The model under review builds one solid part; all positions refer to its coordinate system, in mm. A direction names the side the tool comes from. Give positions to 0.01 mm unless a question says otherwise; leave off trailing zeros. Loops run counter-clockwise (first coordinate to the right, second up) from the corner with the lowest first, then second, coordinate; pieces in that order, holes last. Notation, with made-up numbers: (62, -18.5) -> (99, -18.5) arc R20 cw to (99, 18.5) -> close; hole circle Ø8 at (2.5, -12.75). An arc over 180 degrees is marked (long way). Write each question's results on one line, items separated by ' | '. Start each with the question number.
Q1. Insertion check: pin 1 Ø15 at (y, z) = (-9.5, 33.5) entering from -X; pin 2 Ø12.5 at (x, y) = (41, -12) entering from +Z; pin 3 Ø8 at (y, z) = (7, 55.5) entering from +X; pin 4 Ø1.5 at (x, z) = (-34, 51) entering from -Y. Each pin has a flat end and moves straight along its axis. Give the tip position at first contact, or say it passes through.
Q2. Wall thickness on L1, parallel to X at y = -10, z = 47; L2, parallel to Z at x = -38.5, y = 4.5; L3, parallel to Y at x = -29, z = 59: over which ranges is each line inside the solid? List them lowest first. Write a range as [from, to].
Q3. Machinability: for faces 1 (the face through (-31.75, 0, 39)), 2 (the face through (-19.05, 0, 38)), 3 (the face through (-57.073, -0.557, 6.261)), which of the approach directions +Z, -Z, +X, -X, +Y, -Y give a long, thin tool a straight path to every point of the face, cutting with its end or side? Answer none if there is none.
Q4. We need section A-A (z = 34). Write out the cut boundary in (x, y).
Q5. We need section D-D (y = -7.5). Write out the cut boundary in (x, z).
Q6. We need section C-C (x = 14). Write out the cut boundary in (y, z).
Q7. Mouldability with a two-part tool opening along Y and no side actions: class faces 4 (the face through (41, 0, 12.7)), 5 (the face through (0, 25.4, 11)), 6 (the face through (25.489, -0.251, 52.073)) as released by +Y, released by -Y, zero draft, split by the parting line, or undercut.
Q8. We need section B-B (y = 4.5). Write out the cut boundary in (x, z), plus the area to 3 significant figures.
from build123d import *

# Parameters (mm, degrees)
F1_DEPTH = 25.4
F3_DEPTH = 63.501
F5_DEPTH = 12.7


with BuildPart() as f1:
    # F0 (on Front) → F1 (new body, symmetric)
    with BuildSketch(Plane.XZ):
        Polygon((-31.75, 0), (0, 0), (31.75, 0), (31.75, 63.5), (19.05, 63.5), (19.05, 12.7), (0, 12.7), (-19.05, 12.7), (-19.05, 63.5), (-31.75, 63.5), align=None)
    extrude(amount=F1_DEPTH, both=True)

    # F2 (on face) → F3 (cut, through all)
    with BuildSketch(Plane.YZ.offset(31.75)):
        with BuildLine():
            ThreePointArc((-11.43, 63.5), (0, 52.07), (11.43, 63.5))
            Line((11.43, 63.5), (-11.43, 63.5))
        make_face()
    extrude(amount=-F3_DEPTH, mode=Mode.SUBTRACT)

    # F4 (on face) → F5 (join)
    with BuildSketch(Plane(origin=(0, 0, 0), x_dir=(1, 0, 0), z_dir=(0, 0, -1))):
        with BuildLine():
            ThreePointArc((-31.75, -25.3289327497), (-13.8397398924, -17.9102601076), (-6.4210672503, 0))
            ThreePointArc((-6.4210672503, 0), (-13.8397398924, 17.9102601076), (-31.75, 25.3289327497))
            Line((-31.75, 25.3289327497), (-31.75, -25.3289327497))
        make_face()
        with BuildLine():
            Line((-31.75, -25.3289327497), (-31.75, 25.3289327497))
            ThreePointArc((-31.75, 25.3289327497), (-57.0789327497, 0), (-31.75, -25.3289327497))
        make_face()
        with BuildLine():
            ThreePointArc((57.0789327497, 0), (49.6602601076, 17.9102601076), (31.75, 25.3289327497))
            Line((31.75, 25.3289327497), (31.75, -25.3289327497))
            ThreePointArc((31.75, -25.3289327497), (49.6602601076, -17.9102601076), (57.0789327497, 0))
        make_face()
    extrude(amount=-F5_DEPTH)


solid = f1.part
Output:
1) pin 1: x = -31.75 | pin 2: z = 12.7 | pin 3: x = 31.75 | pin 4: through
2) L1: [-31.75, -19.05], [19.05, 31.75] | L2: [0, 12.7] | L3: [-25.4, -10.51], [10.51, 25.4]
3) face 1: +Z, -X, +Y, -Y | face 2: +Z, +Y, -Y | face 3: +Z, -Z, -X
4) outline: (-31.75, -25.4) -> (-19.05, -25.4) -> (-19.05, 25.4) -> (-31.75, 25.4) -> close; (19.05, -25.4) -> (31.75, -25.4) -> (31.75, 25.4) -> (19.05, 25.4) -> close
5) outline: (-55.94, 0) -> (55.94, 0) -> (55.94, 12.7) -> (31.75, 12.7) -> (31.75, 54.87) -> (19.05, 54.87) -> (19.05, 12.7) -> (-19.05, 12.7) -> (-19.05, 54.87) -> (-31.75, 54.87) -> (-31.75, 12.7) -> (-55.94, 12.7) -> close
6) outline: (-25.4, 0) -> (25.4, 0) -> (25.4, 12.7) -> (-25.4, 12.7) -> close
7) face 4: zero draft | face 5: released by +Y | face 6: undercut
8) outline: (-56.68, 0) -> (56.68, 0) -> (56.68, 12.7) -> (31.75, 12.7) -> (31.75, 52.99) -> (19.05, 52.99) -> (19.05, 12.7) -> (-19.05, 12.7) -> (-19.05, 52.99) -> (-31.75, 52.99) -> (-31.75, 12.7) -> (-56.68, 12.7) -> close | area: 2,460 mm2
